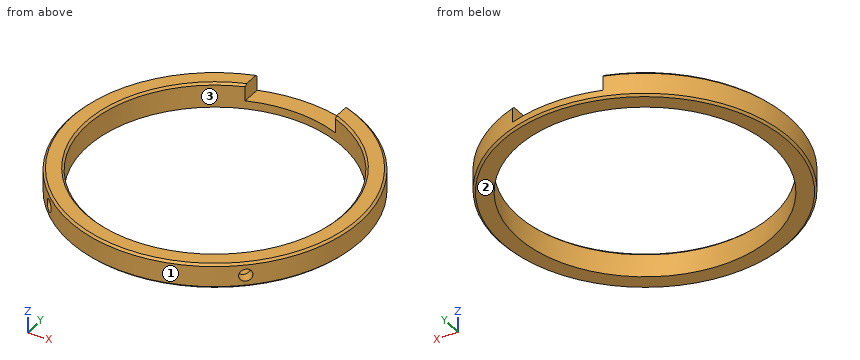
Autodesk Inventor part; units mm, degrees
ref_plane "工作平面1" through (0, 0, 3) normal (0, 0, 1) x (1, 0, 0)
ref_plane "工作平面2" through (24, -26.1582, 3) normal (0.6761, -0.7368, 0) x (0.7368, 0.6761, 0)
ref_plane "工作平面3" through (-24, -26.1582, 3) normal (-0.6761, -0.7368, 0) x (0.7368, -0.6761, 0)
sketch "草圖1" plane through (0, 0, 0) normal (0, 0, 1) x (1, 0, 0)
  circle A0 centre (0, 0) radius 35.5
  circle A1 centre (0, 0) radius 31.15
  dimension "d0" = 71
  dimension "d3" = 62.3
extrude "擠出1" add sketch "草圖1" along normal blind 6
sketch "草圖2" plane through (0, 0, 6) normal (0, 0, 1) x (1, 0, 0)
  circle A0 centre (0, 0) radius 31.15
  circle A1 centre (0, 0) radius 35.5
  line L0 (0, 0) -> (0, 35.5)
  line L1 (11, 33.7528) -> (11, 29.1431)
  line L2 (-11, 33.7528) -> (-11, 29.1431)
  dimension "d6" = 22
extrude "擠出2" cut sketch "草圖2" against normal blind 4 contours A0 L0 A1 L1 | L2 A1 L0 A0
ref_plane "工作平面1" through (0, 0, 3) normal (0, 0, 1) x (1, 0, 0)
sketch "草圖3" plane through (0, 0, 3) normal (0, 0, 1) x (1, 0, 0)
  line L0 (0, 0) -> (0, -42.4806)
  line L1 (0, 0) -> (-24, -26.1582)
  line L2 (0, 0) -> (24, -26.1582)
  arc A0 (-11, 33.7528) -> (11, 33.7528) centre (0, 0) ccw
  line L3 (-24, -26.1582) -> (24, -26.1582)
  dimension "d9" = 48
ref_plane "工作平面2" through (24, -26.1582, 3) normal (0.6761, -0.7368, 0) x (0.7368, 0.6761, 0)
ref_plane "工作平面3" through (-24, -26.1582, 3) normal (-0.6761, -0.7368, 0) x (0.7368, -0.6761, 0)
sketch "草圖4" plane through (24, -26.1582, 3) normal (0.6761, -0.7368, 0) x (0.7368, 0.6761, 0)
  point P0 (0, -3)
  point P1 (0, 0)
hole "孔1" at (24, -26.1582, 3) direction (-0.6761, 0.7368, 0) diameter 3 depth 2.5 tip angle 118
sketch "草圖5" plane through (-24, -26.1582, 3) normal (-0.6761, -0.7368, 0) x (0.7368, -0.6761, 0)
  point P0 (0, -3)
  point P1 (0, 0)
hole "孔2" at (-24, -26.1582, 3) direction (0.6761, 0.7368, 0) diameter 3 depth 2.5 tip angle 118
chamfer "倒角1" distance 0.5 angle 45 5 edges at (-17.7154, -25.622, 6) (25.622, 17.7154, 6) (-35.5, 0, 0) (-20.8537, -28.7293, 6) (28.7293, 20.8537, 6)
properties part number "KE-SP-02-P1"
For this review, take the finished solid that the model builds, in its own axes (mm). Face numbers are marked on the shaded views. Round coordinates to 2 decimals unless told otherwise and drop trailing zeros. Loops run counter-clockwise (first coordinate to the right, second up) from the corner with the lowest first, then second, coordinate; pieces in that order, holes last. Notation, with made-up numbers: (30.5, 67.5) - (89.5, 67.5) arc R15 cw to (89.5, 80.5) - close; hole circle Ø5 at (36, 89.5). An arc over 180 degrees is marked (long way). One line per item, written item: value. Start each with the question number.
Item 1: Take a section at A-A (x = 0). Give the boundary of the cut face in (y, z).
Item 2: For L1, parallel to X at y = 0, z = 2.6; L2, parallel to Y at x = 0, z = 3.1, list the stretches that pass through material, from the lowest coordinate up.
Item 3: The part is to be moulded in two halves that separate along Y. For the marked faces 1, 2 and 3, say which applies: +Y half, -Y half, draft (parallel to the pull), parting line (faces both ways), or undercut.
Item 4: Clearance check with flat-ended pins moving along their axes: pin 1 Ø5 at (x, y) = (2, 33) entering from +Z; pin 2 Ø3 at (y, z) = (31.5, 3) entering from +X; pin 3 Ø1.2 at (y, z) = (30.5, 4) entering from -X. State where each tip first meets the part, or that it passes through.
Item 5: Take a section at B-B (y = 0). Give the boundary of the cut face in (x, z), plus the area to 4 significant figures.
Answer below:
1. outline: (-35.5, 0.5) - (-35, 0) - (-31.15, 0) - (-31.15, 5.5) - (-31.65, 6) - (-35, 6) - (-35.5, 5.5) - close; (31.15, 0) - (35, 0) - (35.5, 0.5) - (35.5, 2) - (31.15, 2) - close
2. L1: x = -35.5 to -31.15, 31.15 to 35.5
2. L2: y = -35.5 to -31.15
3. face 1: parting line
3. face 2: draft
3. face 3: undercut
4. pin 1: stops at z = 2
4. pin 2: stops at x = 18.98
4. pin 3: stops at x = -19.14
5. outline: (-35.5, 0.5) - (-35, 0) - (-31.15, 0) - (-31.15, 5.5) - (-31.65, 6) - (-35, 6) - (-35.5, 5.5) - close; (31.15, 0) - (35, 0) - (35.5, 0.5) - (35.5, 5.5) - (35, 6) - (31.65, 6) - (31.15, 5.5) - close
5. area: 51.45 mm2
